For this review, take the finished solid that the model builds, in its own axes (mm). A direction names the side the tool comes from. Round coordinates to 2 decimals unless told otherwise and drop trailing zeros. Write each loop counter-clockwise with the first axis right and the second up, starting at its lowest first coordinate (ties: lowest second). Pieces come first, ordered by that corner, then holes. Notation, with made-up numbers: (-1.75, -18) - (50.25, -18) arc R36 ccw to (50.25, 19) - close; hole circle Ø3 at (-27.5, -13). An arc over 180 degrees is marked (long way). One line per item, written item: value. Start each with the question number.
Q1. Tool access review of faces 4 (the face through (-0.37, 11.48, 1.66)), 5 (the face through (-4.006, 1.134, -1.262)), 6 (the face through (5.5, -10, 12.7)), 7 (the face through (45.87, 6.088, 29.674)), 8 (the face through (-40.8, 7, 28)): name each direction out of +Z, -Z, +X, -X, +Y, -Y from which nothing blocks a thin tool from reaching the whole face with its end or side.
Q2. Clearance check with flat-ended pins moving along their axes: pin 1 Ø5 at (y, z) = (6, 26.5) entering from -X; pin 2 Ø4 at (y, z) = (6.95, 27.596) entering from +X; pin 3 Ø5.5 at (x, z) = (0, 0) entering from +Y; pin 4 Ø6 at (x, z) = (3.5, 28.5) entering from +Y. State where each tip first meets the part, or that it passes through.
Q3. Add section C-C on x = -25. Write out the cut boundary in (y, z), and give its area (3 significant figures).
Q4. Mouldability with a two-part tool opening along Y and no side actions: class faces 1 (the face through (-2, 2.3, 0)), 2 (the face through (1, 20.4, 2)), 3 (the face through (40.8, 7, 28)) as +Y half, -Y half, draft (parallel to the pull), parting line (faces both ways), or undercut.
Q5. Add section D-D on y = 6.95. Write out the cut boundary in (x, z), and give its area (3 significant figures).
Q6. For probe 1 along Z at (x, y) = (0, 16); probe 2 along Z at (x, y) = (0, 13.5); probe 3 along Y at (x, z) = (-12, 14), list the stretches that pass through material, from the lowest coordinate up.
Q7. Add section B-B on z = 23.56. Write out the cut boundary in (x, y).
Q8. Add section A-A on y = 12.7. Write out the cut boundary in (x, z).
```python
from build123d import *

# Parameters (mm, degrees)
SKETCH1_W                                        = 101.6
SKETCH1_H                                        = 76.2
BOSS_EXTRUDE1_DEPTH                              = 25.4
CBORE_FOR_M3_HEX_HEAD_MACHINE_SCREW1_D           = 3.4
CBORE_FOR_M3_HEX_HEAD_MACHINE_SCREW1_DEPTH       = 25.4
CBORE_FOR_M3_HEX_HEAD_MACHINE_SCREW1_CBORE_D     = 8.4
CBORE_FOR_M3_HEX_HEAD_MACHINE_SCREW1_CBORE_DEPTH = 2.3
SKETCH9_R                                        = 7.5
CUT_EXTRUDE1_DEPTH                               = 5
CUT_EXTRUDE1_TAPER                               = 45
SKETCH12_R                                       = 5
CUT_EXTRUDE3_DEPTH                               = 10
SKETCH13_R                                       = 2.1336
CUT_EXTRUDE4_DEPTH                               = 102.6
CUT_EXTRUDE5_REACH                               = 27.4
SKETCH14_R                                       = 12
SKETCH14_2_R                                     = 14.54
SKETCH14_2_R_2                                   = 12
EXTRUDE_THIN1_DEPTH                              = 10
SKETCH15_R                                       = 2.25
CUT_EXTRUDE6_DEPTH                               = 10


with BuildPart() as part:
    # Sketch1 → Boss-Extrude1 (new body)
    with BuildSketch(Plane(origin=(0, 0, 0), x_dir=(1, 0, 0), z_dir=(0, 1, 0))):
        Rectangle(SKETCH1_W, SKETCH1_H)
    extrude(amount=BOSS_EXTRUDE1_DEPTH)

    # CBORE for M3 Hex Head Machine Screw1
    with Locations(Plane(origin=(0, 0, 0), x_dir=(-1, 0, 0), z_dir=(0, -1, 0))):
        with Locations((0, 0)):
            CounterBoreHole(CBORE_FOR_M3_HEX_HEAD_MACHINE_SCREW1_D / 2, CBORE_FOR_M3_HEX_HEAD_MACHINE_SCREW1_CBORE_D / 2, CBORE_FOR_M3_HEX_HEAD_MACHINE_SCREW1_CBORE_DEPTH, depth=CBORE_FOR_M3_HEX_HEAD_MACHINE_SCREW1_DEPTH)

    # Sketch9 → Cut-Extrude1 (cut)
    with BuildSketch(Plane(origin=(0, 25.4, 0), x_dir=(1, 0, 0), z_dir=(0, 1, 0))):
        Circle(SKETCH9_R)
    extrude(amount=-CUT_EXTRUDE1_DEPTH, taper=CUT_EXTRUDE1_TAPER, mode=Mode.SUBTRACT)

    # Sketch12 → Cut-Extrude3 (cut)
    with BuildSketch(Plane(origin=(0, 25.4, 0), x_dir=(1, 0, 0), z_dir=(0, 1, 0))):
        with Locations((0, -20)):
            Circle(SKETCH12_R)
    extrude(amount=-CUT_EXTRUDE3_DEPTH, mode=Mode.SUBTRACT)

    # Sketch13 → Cut-Extrude4 (cut, through all)
    with BuildSketch(Plane.ZY.offset(50.8)):
        with Locations((-6.604, 12.7)):
            Circle(SKETCH13_R)
    extrude(amount=-CUT_EXTRUDE4_DEPTH, mode=Mode.SUBTRACT)

    # Sketch14 → Cut-Extrude5 (cut, up to next)
    with BuildSketch(Plane(origin=(0, 0, 0), x_dir=(-1, 0, 0), z_dir=(0, -1, 0)), mode=Mode.PRIVATE) as cut_extrude5_sk1:
        with Locations((0, -23.56)):
            Circle(SKETCH14_R)
    cut_extrude5_tool1 = extrude(cut_extrude5_sk1.sketch, amount=-CUT_EXTRUDE5_REACH, mode=Mode.PRIVATE) & part.part
    add(cut_extrude5_tool1.solids().sort_by_distance((0, 0, 23.56))[0], mode=Mode.SUBTRACT)

    # Sketch14<2> → Extrude-Thin1 (add)
    with BuildSketch(Plane(origin=(0, 0, 0), x_dir=(-1, 0, 0), z_dir=(0, -1, 0))):
        with Locations((0, -23.56)):
            Circle(SKETCH14_2_R)
        with Locations((0, -23.56)):
            Circle(SKETCH14_2_R_2, mode=Mode.SUBTRACT)
    extrude(amount=EXTRUDE_THIN1_DEPTH)

    # Sketch15 → Cut-Extrude6 (cut)
    with BuildSketch(Plane.ZY.offset(50.8)):
        with Locations((27.596, 6.95)):
            Circle(SKETCH15_R)
    cut_extrude6 = extrude(amount=-CUT_EXTRUDE6_DEPTH, mode=Mode.SUBTRACT)

    # Mirror1: Cut-Extrude6 across plane
    add(cut_extrude6.mirror(Plane(origin=(0, 0, 0), x_dir=(0, 0, 1), z_dir=(1, 0, 0))), mode=Mode.SUBTRACT)


solid = part.part
```
Result set:
1. face 4: +Y, -Y
1. face 5: -Y
1. face 6: +Z, -Z, +X, -X, -Y
1. face 7: +X
1. face 8: -X
2. pin 1: stops at x = -50.8
2. pin 2: stops at x = 40.8
2. pin 3: stops at y = 20.65
2. pin 4: passes through
3. outline: (0, -38.1) - (25.4, -38.1) - (25.4, 38.1) - (0, 38.1) - close; hole circle Ø4.27 at (12.7, -6.6)
3. area: 1,920 mm^2
4. face 1: -Y half
4. face 2: +Y half
4. face 3: undercut
5. outline: (-50.8, -38.1) - (50.8, -38.1) - (50.8, 25.35) - (40.8, 25.35) - (40.8, 29.85) - (50.8, 29.85) - (50.8, 38.1) - (-50.8, 38.1) - (-50.8, 29.85) - (-40.8, 29.85) - (-40.8, 25.35) - (-50.8, 25.35) - close; hole circle Ø24 at (0, 23.56); hole circle Ø3.4 at (0, 0)
5. area: 7,190 mm^2
6. probe 1: z = -38.1 to -1.7, 1.7 to 11.56, 35.56 to 38.1
6. probe 2: z = -38.1 to -8.58, -4.63 to -1.7, 1.7 to 11.56, 35.56 to 38.1
6. probe 3: y = 0 to 25.4
7. outline: (-50.8, 0) - (-14.54, 0) - (-14.54, -10) - (-12, -10) - (-12, 25.4) - (-50.8, 25.4) - close; (12, -10) - (14.54, -10) - (14.54, 0) - (50.8, 0) - (50.8, 25.4) - (12, 25.4) - close
8. outline: (-50.8, -38.1) - (50.8, -38.1) - (50.8, -8.74) - (-50.8, -8.74) - close; (-50.8, -4.47) - (50.8, -4.47) - (50.8, 38.1) - (-50.8, 38.1) - close; hole circle Ø24 at (0, 23.56); hole circle Ø3.4 at (0, 0)
